from build123d import *

# Parameters (mm, degrees)
F1_DEPTH = 25.4
F2_R     = 5.08
F3_R     = 6.157745
F3_W     = 0.458606
F3_H     = 2.747152
F3_R_2   = 4.937025
F4_DEPTH = 25.4


with BuildPart() as f1:
    # F0 (on Right) → F1 (new body)
    with BuildSketch(Plane.YZ):
        Polygon((1.631016, 33.007801), (-38.663846, 33.007801), (-38.663846, 20.186709), (70.824213, 20.186709), (70.824213, 43.99731), (55.357497, 43.99731), (1.631016, 43.99731), align=None)
    extrude(amount=F1_DEPTH)

    # F2
    f2_edges = [f1.edges().sort_by_distance(p)[0] for p in [
        (25.4, 36.227615, 43.99731),
        (25.4, -18.516415, 33.007801),
        (12.7, 1.631016, 43.99731),
        (0, -18.516415, 33.007801),
        (25.4, -38.663846, 26.597255),
        (0, -38.663846, 26.597255),
        (25.4, 16.080184, 20.186709),
        (0, 16.080184, 20.186709),
        (0, 70.824213, 32.09201),
        (0, 36.227615, 43.99731),
        (0, 1.631016, 38.502555),
        (12.7, 70.824213, 20.186709),
        (12.7, 70.824213, 43.99731),
        (25.4, 70.824213, 32.09201),
    ]]
    fillet(f2_edges, radius=F2_R)

    # F3 (on face) → F4 (join)
    with BuildSketch(Plane.YZ.offset(25.4)):
        with Locations((56.599278, 32.443203)):
            Circle(F3_R)
        with Locations((56.828581, 31.069627)):
            Rectangle(F3_W, F3_H, mode=Mode.SUBTRACT)
        with Locations((7.300105, 30.641174)):
            Circle(F3_R_2)
    extrude(amount=-F4_DEPTH)


solid = f1.part
The model under review builds one solid part; all positions refer to its coordinate system, in mm. A direction names the side the tool comes from. Give positions to 0.01 mm unless a question says otherwise; leave off trailing zeros. Loops run counter-clockwise (first coordinate to the right, second up) from the corner with the lowest first, then second, coordinate; pieces in that order, holes last. Notation, with made-up numbers: (59.25, 19.5) -> (118.25, 19.5) arc R22 ccw to (118.25, 55.5) -> close; hole circle Ø7 at (27, 81.25). An arc over 180 degrees is marked (long way). Answer as a JSON object with one key per item and string values. Group by question number.
Q1. Tool access review of faces 1 (the cylindrical face through (2.21, 2.52, 36.2)), 2 (the flat face through (13, -18, 33.008)), 3 (the flat face through (13, 37, 43.997)): name each direction out of +Z, -Z, +X, -X, +Y, -Y from which nothing blocks a thin tool from reaching the whole face with its end or side.
Q2. Take a section at B-B (x = 18.25). Write out the cut boundary in (y, z).
Q3. Take a section at C-C (z = 41). Write out the cut boundary in (x, y), plus the area to 3 significant figures.
Q4. Insertion check: pin 1 (4 mm diameter, centred on y = -13.5, z = 30.5, fed in from -X); pin 2 (5 mm diameter, centred on x = 3, y = -15.5, fed in from +Z); pin 3 (8 mm diameter, centred on y = -2.5, z = 36, fed in from +X). Each pin has a flat end and moves straight along its axis. Give the tip position at first contact, or say it passes through.
Q5. Take a section at A-A (y = 34). Write out the cut boundary in (x, z), plus the area to 3 significant figures.
Q6. Take a section at D-D (y = -28). Write out the cut boundary in (x, z).
Q7. Wall thickness on line 1 along Y through (x, z) = (12, 36); line 2 along Z through (x, y) = (15.5, -12); line 3 along Z through (x, y) = (12.5, 66): over which ranges is each line inside the solid? List them lowest first.
Answer below:
{
 "1": {"face 1": "+Z, -X, -Y", "face 2": "+Z, +X, -X, -Y", "face 3": "+Z, +X, -X, +Y, -Y"},
 "2": {"outline": "(-38.66, 20.19) -> (65.74, 20.19) arc R5.08 ccw to (70.82, 25.27) -> (70.82, 38.92) arc R5.08 ccw to (65.74, 44) -> (6.71, 44) arc R5.08 ccw to (1.63, 38.92) -> (1.63, 33.01) -> (-38.66, 33.01) -> close"},
 "3": {"outline": "(0.45, 6.71) arc R4.63 ccw to (5.08, 2.08) -> (24.95, 2.08) -> (24.95, 65.74) arc R4.63 ccw to (20.32, 70.38) -> (5.08, 70.38) arc R4.63 ccw to (0.45, 65.74) -> close", "area": "1,660 mm2"},
 "4": {"pin 1": "stops at x = 0.03", "pin 2": "stops at z = 33.01", "pin 3": "stops at x = 23.36"},
 "5": {"outline": "(0, 25.27) arc R5.08 ccw to (5.08, 20.19) -> (20.32, 20.19) arc R5.08 ccw to (25.4, 25.27) -> (25.4, 38.92) arc R5.08 ccw to (20.32, 44) -> (5.08, 44) arc R5.08 ccw to (0, 38.92) -> close", "area": "583 mm2"},
 "6": {"outline": "(0, 25.27) arc R5.08 ccw to (5.08, 20.19) -> (20.32, 20.19) arc R5.08 ccw to (25.4, 25.27) -> (25.4, 27.93) arc R5.08 ccw to (20.32, 33.01) -> (5.08, 33.01) arc R5.08 ccw to (0, 27.93) -> close"},
 "7": {"line 1": "y = 1.63 to 70.82", "line 2": "z = 20.19 to 33.01", "line 3": "z = 20.19 to 43.99"}
}
